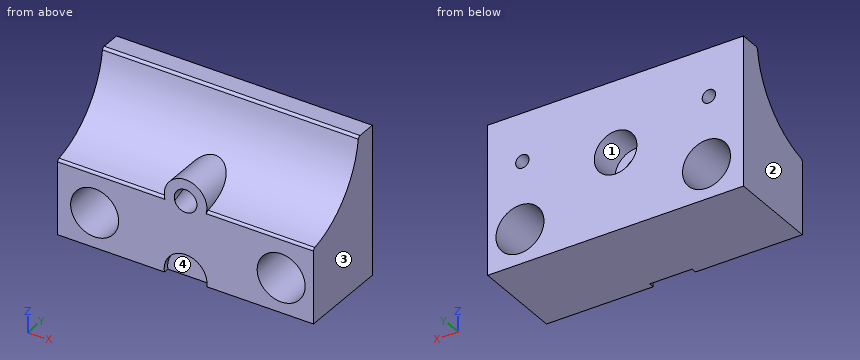
from build123d import *

# Parameters (mm, degrees)
F1_DEPTH      = 152.4
F2_R          = 14.2875
F3_DEPTH      = 101.6
F4_R          = 12.7
F4_R_2        = 6.746875
F5_DEPTH      = 19.05
F6_DEPTH      = 76.2
F7_DEPTH      = 34.925
F8_R          = 12.7653078778
F9_DEPTH      = 3.175
F10_T1_DEPTH  = 159.4216090421
F10_T6_DEPTH  = 70.1643898363
F10_S7_R      = 12.7
F10_T8_DEPTH  = 37
F10_T12_DEPTH = 70.1643898363
F10_S13_R     = 12.7
F10_T14_DEPTH = 37
F11_R         = 3.96875
F12_DEPTH     = 12.7


# Not quite as in the source:
# - a fillet or chamfer that OpenCascade refuses, or shapes differently, is made with other operations: its cross-section is extruded or revolved along the edge and cut away or added
# - a length typed as a fraction of an inch, garbled in the dataset ("3 / 203.2 mm" for 3/8 in), is restored


with BuildPart() as f1:
    # F0 (on Right) → F1 (new body)
    with BuildSketch(Plane.YZ):
        with BuildLine():
            Line((-53.975, 44.45), (-53.975, 0))
            Line((-53.975, 0), (0, 0))
            Line((0, 0), (0, 88.9))
            Line((0, 88.9), (-12.7, 88.9))
            ThreePointArc((-12.7, 88.9), (-25.9749076509, 59.8383071044), (-53.975, 44.45))
        make_face()
    extrude(amount=-F1_DEPTH)

    # F2 (on face) → F3 (cut)
    with BuildSketch(Plane.XZ.offset(53.975)):
        with Locations((-130.3763389587, 20.6375)):
            Circle(F2_R)
        with Locations((-19.2513389587, 20.6375)):
            Circle(F2_R)
    extrude(amount=-F3_DEPTH, mode=Mode.SUBTRACT)

    # F4 (on face) → F5 (cut)
    with BuildSketch(Plane(origin=(0, 0, 0), x_dir=(-1, 0, 0), z_dir=(0, 1, 0))):
        with Locations((76.2, 46.355)):
            Circle(F4_R)
        with Locations((76.2, 46.355)):
            Circle(F4_R_2, mode=Mode.SUBTRACT)
    extrude(amount=-F5_DEPTH, mode=Mode.SUBTRACT)

    # F6 (cut): a face of the model
    f6_faces = [f1.faces().sort_by_distance(p)[0] for p in [
        (-76.2, 0, 46.355),
    ]]
    extrude(f6_faces, amount=-F6_DEPTH, mode=Mode.SUBTRACT)

    # F7 (add, through all): a face of the model
    f7_faces = [f1.faces().sort_by_distance(p)[0] for p in [
        (-63.8592102448, -19.05, 46.355),
    ]]
    extrude(f7_faces, amount=-F7_DEPTH)

    # F8 (on face) → F9 (cut)
    with BuildSketch(Plane.XZ.offset(53.975)):
        with Locations((-76.2, 1.905)):
            Circle(F8_R)
    extrude(amount=-F9_DEPTH, mode=Mode.SUBTRACT)

    # F10: fillet of radius 1.5875 on 3 edges, made by hand

    # F10_s2 → F10_t1 (cut)
    with BuildSketch(Plane.YZ.offset(-155.9108045211)):
        with BuildLine():
            ThreePointArc((-12.8685611865, 87.5274309986), (-12.3394581707, 88.5086101977), (-11.2956781916, 88.9))
            Line((-11.2956781916, 88.9), (-12.7, 88.9))
            ThreePointArc((-12.7, 88.9), (-12.7796098579, 88.2131418999), (-12.8685611865, 87.5274309986))
        make_face()
    extrude(amount=F10_T1_DEPTH, mode=Mode.SUBTRACT)


with BuildPart() as f10_tool4:
    # F10_s5 → F10_t6 (new body)
    with BuildSketch(Plane.YZ.offset(-85.4959611607)):
        with BuildLine():
            ThreePointArc((-52.7151762735, 44.6991736422), (-53.6204522161, 44.1458521426), (-53.975, 43.1458596012))
            Line((-53.975, 43.1458596012), (-53.975, 44.45))
            ThreePointArc((-53.975, 44.45), (-53.3443007137, 44.5706056045), (-52.7151762735, 44.6991736422))
        make_face()
    extrude(amount=-F10_T6_DEPTH)

    # F10_s7 → F10_t8 (cut, symmetric)
    with BuildSketch(Plane.XZ.offset(53.3)):
        with Locations((-76.2, 46.355)):
            Circle(F10_S7_R)
    extrude(amount=F10_T8_DEPTH, both=True, mode=Mode.SUBTRACT)


with BuildPart() as f1_1:
    add(f1.part)

    # F10_t3: cut F10_tool4
    add(f10_tool4.part, mode=Mode.SUBTRACT)


with BuildPart() as f10_tool10:
    # F10_s11 → F10_t12 (new body)
    with BuildSketch(Plane.YZ.offset(3.2603509969)):
        with BuildLine():
            ThreePointArc((-52.7151762735, 44.6991736422), (-53.6204522161, 44.1458521426), (-53.975, 43.1458596012))
            Line((-53.975, 43.1458596012), (-53.975, 44.45))
            ThreePointArc((-53.975, 44.45), (-53.3443007137, 44.5706056045), (-52.7151762735, 44.6991736422))
        make_face()
    extrude(amount=-F10_T12_DEPTH)

    # F10_s13 → F10_t14 (cut, symmetric)
    with BuildSketch(Plane.XZ.offset(53.3)):
        with Locations((-76.2, 46.355)):
            Circle(F10_S13_R)
    extrude(amount=F10_T14_DEPTH, both=True, mode=Mode.SUBTRACT)


with BuildPart() as f1_2:
    add(f1_1.part)

    # F10_t9: cut F10_tool10
    add(f10_tool10.part, mode=Mode.SUBTRACT)

    # F11 (on face) → F12 (cut)
    with BuildSketch(Plane(origin=(0, 0, 0), x_dir=(-1, 0, 0), z_dir=(0, 1, 0))):
        with Locations((20.6375, 60.325)):
            Circle(F11_R)
        with Locations((131.7625, 60.325)):
            Circle(F11_R)
    extrude(amount=-F12_DEPTH, mode=Mode.SUBTRACT)


solid = f1_2.part
Could you check a few things on this model? Use its own coordinates, in mm. Face numbers are marked on the shaded views. Give positions to 0.01 mm unless a question says otherwise; leave off trailing zeros. Order: outer loops, then holes, each group sorted by start corner. A loop starts at its lowest first (then second) coordinate and runs counter-clockwise, first axis right, second up.
1. Will these pins go through, and if not, where does the flat tip stop? P1, Ø2.5, axis at x = -131.5, z = 62, coming from the +Y side; P2, Ø8, axis at x = -62, z = 78.5, coming from the -Y side; P3, Ø12.5, axis at x = -75.5, z = 49.5, coming from the +Y side; P4, Ø11, axis at x = -76.2, z = 46.355, coming from the +Y side.
2. Suppose I cut it at C-C (y = -23.5). List the corners of the cut face in (x, z) for me (1 decimal).
3. I need wall thicknesses on L1, parallel to X at y = -36.5, z = 27; L2, parallel to Z at x = -134, y = -5; L3, parallel to X at y = -4, z = 48. Which ranges of each line are inside material? Lowest first, please.
4. We'd pull the mould along X, two halves only. Please class the marked faces 1, 2, 3 and 4: pulls with the +X half, pulls with the -X half, needs draft (parallel to the pull), parting line crosses it, or undercut.
5. Suppose I cut it at B-B (z = 30.5). List the corners of the cut face in (x, y) for me (3 decimals), plus the area to 3 significant figures.
6. Suppose I cut it at D-D (x = -45). List the corners of the cut face in (y, z) for me (1 decimal), plus the area to 3 significant figures.
Solved:
1. P1: stops at y = -12.7
1. P2: stops at y = -16.46
1. P3: stops at y = -19.05
1. P4: passes through
2. outline: (-152.4, 0) - (0, 0) - (0, 62.7) - (-152.4, 62.7) - close; hole circle Ø28.6 at (-130.4, 20.6); hole circle Ø13.5 at (-76.2, 46.4); hole circle Ø28.6 at (-19.3, 20.6)
3. L1: x = -152.4 to -143.17, -117.58 to -32.04, -6.46 to 0
3. L2: z = 0 to 6.82, 34.46 to 57.05, 63.6 to 88.9
3. L3: x = -152.4 to -88.79, -63.61 to 0
4. face 1: undercut
4. face 2: pulls with the -X half
4. face 3: pulls with the +X half
4. face 4: undercut
5. outline: (-152.4, -53.975) - (-140.714, -53.975) - (-140.714, 0) - (-152.4, 0) - close; (-120.039, -53.975) - (-29.589, -53.975) - (-29.589, 0) - (-120.039, 0) - close; (-8.914, -53.975) - (0, -53.975) - (0, 0) - (-8.914, 0) - close
5. area: 5,990 mm2
6. outline: (-54, 0) - (0, 0) - (0, 88.9) - (-11.3, 88.9) arc R1.6 ccw to (-12.9, 87.5) arc R50.8 cw to (-52.7, 44.7) arc R1.6 ccw to (-54, 43.1) - close
6. area: 3,470 mm2
